Can you work these out from the model? Positions are in its coordinate system, mm. A direction names the side the tool comes from. Round coordinates to 2 decimals unless told otherwise and drop trailing zeros. Order: outer loops, then holes, each group sorted by start corner. A loop starts at its lowest first (then second) coordinate and runs counter-clockwise, first axis right, second up. Notation, with made-up numbers: M 22.25,48.25 L 33.25,48.25 A18 cw 33.25,57.25 Z; hole C -29.75,9 d6. An arc over 180 degrees is marked long. Answer as a JSON object with one key per item and string values. Group by question number.
```python
from build123d import *

# Parameters (mm, degrees)
SKETCH_W    = 45
SKETCH_H    = 39
SKETCH_R    = 2
SKETCH_W_2  = 21.5
SKETCH_H_2  = 29
PAD_DEPTH   = 4
FILLET_R    = 6
FILLET001_R = 6
FILLET002_R = 1


with BuildPart() as part:
    # Sketch → Pad (new body)
    with BuildSketch(Plane.XY):
        with Locations((17.5, 14.5)):
            Rectangle(SKETCH_W, SKETCH_H)
        with Locations((33.5, 2)):
            Circle(SKETCH_R, mode=Mode.SUBTRACT)
        with Locations((33.5, 27)):
            Circle(SKETCH_R, mode=Mode.SUBTRACT)
        with Locations((10.75, 14.5)):
            Rectangle(SKETCH_W_2, SKETCH_H_2, mode=Mode.SUBTRACT)
    extrude(amount=PAD_DEPTH)

    # Fillet
    fillet_edges = [part.edges().sort_by_distance(p)[0] for p in [
        (40, -5, 2),
        (-5, -5, 2),
    ]]
    fillet(fillet_edges, radius=FILLET_R)

    # Fillet001
    fillet001_edges = [part.edges().sort_by_distance(p)[0] for p in [
        (-5, 34, 2),
        (40, 34, 2),
    ]]
    fillet(fillet001_edges, radius=FILLET001_R)

    # Fillet002
    fillet002_edges = [part.edges().sort_by_distance(p)[0] for p in [
        (0, 29, 2),
        (0, 0, 2),
        (21.5, 0, 2),
        (21.5, 29, 2),
    ]]
    fillet(fillet002_edges, radius=FILLET002_R)


solid = part.part
```
1) I need wall thicknesses on line 1 along Y through (x, z) = (33.5, 2.3); line 2 along X through (y, z) = (28, 1.7); line 3 along X through (y, z) = (2.5, 2). Which ranges of each line are inside material? Lowest first, please.
2) If we section it at A-A on x = 33.5: Write out the boundary of the cut face in (y, z).
3) Which directions (+Z, -Z, +X, -X, +Y, -Y) give clear straight access to the entire face, cutting with the end or side of a thin tool? Please do faces 1 (the face through (11, 0, 2)), 2 (the face through (22, 15, 0)).
4) If we section it at D-D on z = 0.5: Write out the boundary of the cut face in (x, y), plus the area to 3 significant figures.
5) For pin 1 (1.5 mm diameter, centred on x = 2, y = 2, fed in from +Z), with a flat end and sliding along its axis, tell me the tip position at first contact or that it passes through.
6) If we section it at C-C on y = 27: Write out the boundary of the cut face in (x, z).
7) If we section it at B-B on y = 20: Write out the boundary of the cut face in (x, z).
Findings:
{
 "1": {"line 1": "y = -5 to 0, 4 to 25, 29 to 34", "line 2": "x = -5 to 0, 21.5 to 31.77, 35.23 to 40", "line 3": "x = -5 to 0, 21.5 to 31.56, 35.44 to 40"},
 "2": {"outline": "M -5,0 L 0,0 L 0,4 L -5,4 Z; M 4,0 L 25,0 L 25,4 L 4,4 Z; M 29,0 L 34,0 L 34,4 L 29,4 Z"},
 "3": {"face 1": "+Z, -Z", "face 2": "-Z, +X, -X, +Y, -Y"},
 "4": {"outline": "M -5,1 A6 ccw 1,-5 L 34,-5 A6 ccw 40,1 L 40,28 A6 ccw 34,34 L 1,34 A6 ccw -5,28 Z; hole M 0,1 A1 ccw 1,0 L 20.5,0 A1 ccw 21.5,1 L 21.5,28 A1 ccw 20.5,29 L 1,29 A1 ccw 0,28 Z; hole C 33.5,2 d4; hole C 33.5,27 d4", "area": "1,080 mm^2"},
 "5": {"pin 1": "passes through"},
 "6": {"outline": "M -5,0 L 0,0 L 0,4 L -5,4 Z; M 21.5,0 L 31.5,0 L 31.5,4 L 21.5,4 Z; M 35.5,0 L 40,0 L 40,4 L 35.5,4 Z"},
 "7": {"outline": "M -5,0 L 0,0 L 0,4 L -5,4 Z; M 21.5,0 L 40,0 L 40,4 L 21.5,4 Z"}
}
